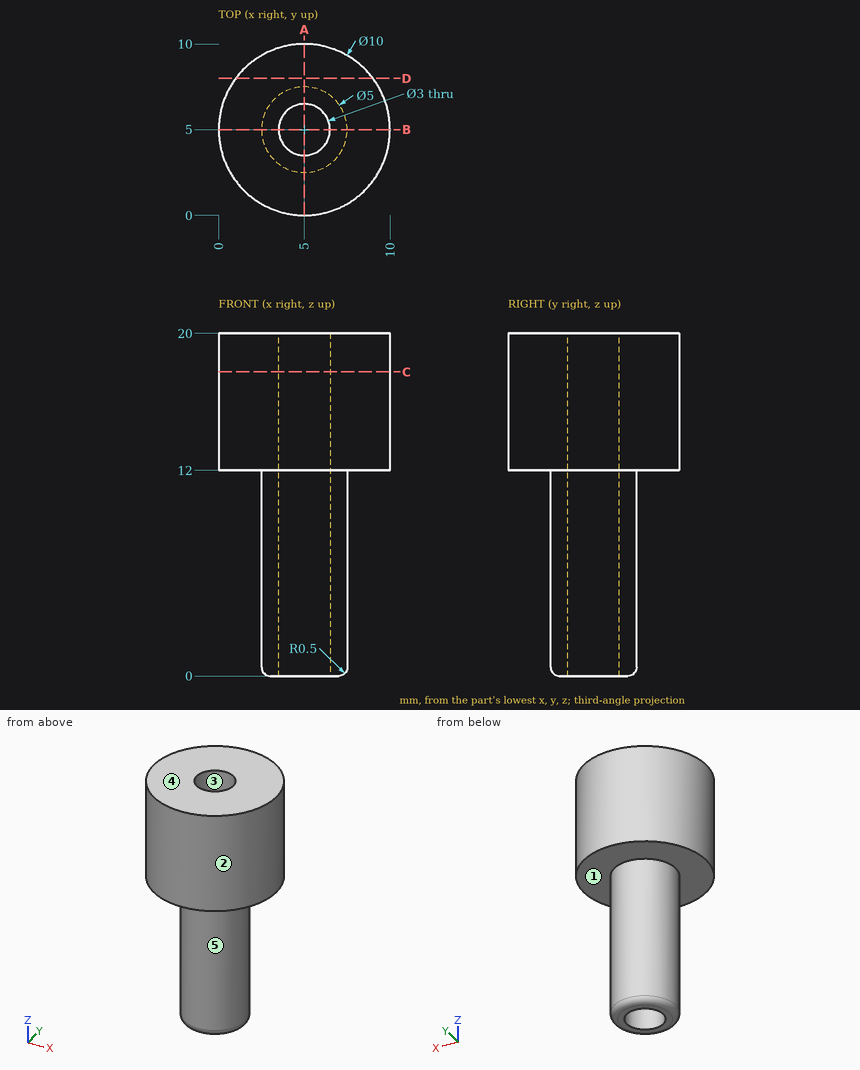
Geometry: see drawing. Coordinates: mm, zero at the bounding-box minimum. A direction names the side the tool comes from. Round coordinates to 2 decimals unless told otherwise and drop trailing zeros. Write each loop counter-clockwise with the first axis right and the second up, starting at its lowest first coordinate (ties: lowest second). Pieces come first, ordered by that corner, then holes.
1) Cut plane D-D (y = 8). Return the cut outline in (x, z).
2) Draft query along X for the marked faces 1, 2 and 3. Return one class per face: pulls with the +X half, pulls with the -X half, needs draft (parallel to the pull), parting line crosses it, or undercut.
3) Reachability of the marked faces 4 and 5 from +Z, -Z, +X, -X, +Y, -Y: full face, straight path, thin tool, end or side. Return the list, or none.
4) Cut plane C-C (z = 17.75). Return the cut outline in (x, y), then the cut area to 3 significant figures.
5) Cut plane A-A (x = 5). Return the cut outline in (y, z), then the cut area to 3 significant figures.
6) Ray query, L1, parallel to Y at x = 5, z = 9.25; L2, parallel to Z at x = 2.75, y = 2.75; L3, parallel to Y at x = 5, z = 14.5. Return the intervals inside material, ascending.
7) Contact query for flat-ended pins moving along their axis: P1, Ø3, axis at y = 7, z = 16.5, coming from the +X side; P2, Ø3, axis at x = 1, z = 15, coming from the -Y side; P3, Ø1.5, axis at x = 7.5, z = 14.5, coming from the -Y side; P4, Ø4, axis at x = 8.5, y = 9, coming from the +Z side. Output: stop coordinate, or through.
Geometry says:
1. outline: (1, 12) - (9, 12) - (9, 20) - (1, 20) - close
2. face 1: needs draft
2. face 2: parting line crosses it
2. face 3: undercut
3. face 4: +Z, +X, -X, +Y, -Y
3. face 5: -Z
4. outline: circle Ø10 at (5, 5); hole circle Ø3 at (5, 5)
4. area: 71.5 mm2
5. outline: (0, 12) - (2.5, 12) - (2.5, 0.5) arc R0.5 ccw to (3, 0) - (3.5, 0) - (3.5, 20) - (0, 20) - close; (6.5, 0) - (7, 0) arc R0.5 ccw to (7.5, 0.5) - (7.5, 12) - (10, 12) - (10, 20) - (6.5, 20) - close
5. area: 79.9 mm2
6. L1: y = 2.5 to 3.5, 6.5 to 7.5
6. L2: z = 12 to 20
6. L3: y = 0 to 3.5, 6.5 to 10
7. P1: stops at x = 9.97
7. P2: stops at y = 0.67
7. P3: stops at y = 0.32
7. P4: stops at z = 20
